For this review, take the finished solid that the model builds, in its own axes (mm). A direction names the side the tool comes from. Give positions to 0.01 mm unless a question says otherwise; leave off trailing zeros. Order: outer loops, then holes, each group sorted by start corner. A loop starts at its lowest first (then second) coordinate and runs counter-clockwise, first axis right, second up. Notation, with made-up numbers: M -35.75,14.5 L -30.75,14.5 A31 cw -30.75,42.5 Z; hole C 24.5,2 d1. An arc over 180 degrees is marked long. Answer as CSV lines item,"result". Start each with the question number.
1. Machinability: for faces 5 (the flat face through (-61, 100, 60)), 6 (the flat face through (24, 25, 12)), which of the approach directions +Z, -Z, +X, -X, +Y, -Y give a long, thin tool a straight path to every point of the face, cutting with its end or side? Answer none if there is none.
2. We need section A-A, the plane x = 0. Give the boundary of the cut face in (y, z), and give its area (3 significant figures).
3. We need section B-B, the plane y = 81.5. Give the boundary of the cut face in (x, z) (3 decimals).
4. Clearance check with flat-ended pins moving along their axes: P1, Ø10, axis at x = 54, y = 39, coming from the +Z side; P2, Ø1.5, axis at x = 19.5, y = 42, coming from the -Z side; P3, Ø2, axis at x = 56, y = 71.5, coming from the -Z side; P4, Ø1, axis at y = 82, z = -16, coming from the +X side. State where each tip first meets the part, or that it passes through.
5. We need section C-C, the plane y = 70. Give the boundary of the cut face in (x, z), and give its area (3 significant figures).
6. For line 1 along Z through (x, y) = (0, 18.5) (3 decimals); line 2 along Z through (x, y) = (0, 10); line 3 along Y through (x, z) = (42, -12.5), list the stretches that pass through material, from the lowest coordinate up.
7. Mouldability with a two-part tool opening along X and no side actions: class faces 1 (the flat face through (-61, 100, -61)), 2 (the conical face through (75.86, 28.48, 31.45)), 3 (the cylindrical face through (-0.55, 75.006, -82.375)), 4 (the cylindrical face through (-0.55, 75.006, 82.774)) as pulls with the +X half, pulls with the -X half, needs draft (parallel to the pull), parting line crosses it, or undercut.
8. We need section D-D, the plane y = 59. Give the boundary of the cut face in (x, z), and give its area (3 significant figures).
from build123d import *

# Parameters (mm, degrees)
SKETCH2_R               = 25
CUT_EXTRUDE2_DEPTH      = 30
CUT_EXTRUDE3_DEPTH      = 174.205080757
CUT_EXTRUDE3_DEPTH_BACK = 174.205080757
SKETCH3_R               = 25
SKETCH4_R               = 25
CUT_EXTRUDE4_DEPTH      = 100


with BuildPart() as part:
    # Sketch1 → Revolve1 (revolve)
    with BuildSketch(Plane.XY):
        Polygon((0, 0), (75, 0), (100, 100), (75, 100), (56.25, 25), (0, 25), align=None)
    revolve(axis=Axis((0, 0, 0), (0, 1, 0)))

    # Sketch2 → Cut-Extrude2 (cut)
    with BuildSketch(Plane(origin=(0, 25, 0), x_dir=(1, 0, 0), z_dir=(0, 1, 0))):
        with Locations(Location((0, 0, 0), (0, 0, 180))):
            Circle(SKETCH2_R)
    extrude(amount=-CUT_EXTRUDE2_DEPTH, mode=Mode.SUBTRACT)

    # Sketch3 → Cut-Extrude3 (cut, two sides: drawn at the far end of the back side and taken through both)
    with BuildSketch(Plane(origin=(0, 0, 0), x_dir=(0, 0, -1), z_dir=(1, 0, 0)).offset(-CUT_EXTRUDE3_DEPTH_BACK)):
        with Locations((0, 100)):
            Circle(SKETCH3_R)
    extrude(amount=CUT_EXTRUDE3_DEPTH + CUT_EXTRUDE3_DEPTH_BACK, mode=Mode.SUBTRACT)

    # Sketch4 → Cut-Extrude4 (cut, symmetric)
    with BuildSketch(Plane.XY):
        with Locations((0, 100)):
            Circle(SKETCH4_R)
    extrude(amount=CUT_EXTRUDE4_DEPTH, both=True, mode=Mode.SUBTRACT)


solid = part.part
Result set:
1,face 5,"+Z, -Z, +X, -X, +Y"
1,face 6,"+Y"
2,outline,"M 0,-75 L 75,-93.75 L 75,-68.75 L 25,-56.25 L 25,-25 L 0,-25 Z; M 0,25 L 25,25 L 25,56.25 L 75,68.75 L 75,93.75 L 0,75 Z"
2,area,"5,160 mm2"
3,outline,"M -93.881,-16.815 A95.375 ccw -16.815,-93.881 L -16.815,-68.337 A70.375 cw -68.337,-16.815 Z; M -93.881,16.815 L -68.337,16.815 A70.375 cw -16.815,68.337 L -16.815,93.881 A95.375 ccw Z; M 16.815,-93.881 A95.375 ccw 93.881,-16.815 L 68.337,-16.815 A70.375 cw 16.815,-68.337 Z; M 16.815,68.337 A70.375 cw 68.337,16.815 L 93.881,16.815 A95.375 ccw 16.815,93.881 Z"
4,P1,"z = 69.47"
4,P2,"z = -83.51"
4,P3,"z = -74.9"
4,P4,"through"
5,outline,"C 0,0 d185; hole C 0,0 d135"
5,area,"12,600 mm2"
6,line 1,"-79.625 to -25, 25 to 79.625"
6,line 2,"-77.5 to -25, 25 to 77.5"
6,line 3,"0 to 25"
7,face 1,"needs draft"
7,face 2,"parting line crosses it"
7,face 3,"undercut"
7,face 4,"undercut"
8,outline,"C 0,0 d179.5; hole C 0,0 d129.5"
8,area,"12,100 mm2"
